Here's how the part is built. I have some questions about the finished solid (model axes, mm). A direction names the side the tool comes from. Give positions to 0.01 mm unless a question says otherwise; leave off trailing zeros. Loops run counter-clockwise (first coordinate to the right, second up) from the corner with the lowest first, then second, coordinate; pieces in that order, holes last. Notation, with made-up numbers: (46, 57) - (73, 57) arc R11 cw to (73, 73) - close; hole circle Ø7 at (18.25, 38). An arc over 180 degrees is marked (long way). Put each result on its own line as item: value. Start each with the question number.
from build123d import *

# Parameters (mm, degrees)
F0_W     = 190.5
F0_H     = 101.6
F0_W_2   = 76.2
F0_H_2   = 76.2
F1_DEPTH = 127
F2_DEPTH = 6.35
F3_R     = 5.08


with BuildPart() as f1:
    # F0 (on Top) → F1 (new body)
    with BuildSketch(Plane.XY):
        Rectangle(F0_W, F0_H)
        with Locations((-44.45, 0)):
            Rectangle(F0_W_2, F0_H_2, mode=Mode.SUBTRACT)
        with Locations((44.45, 0)):
            Rectangle(F0_W_2, F0_H_2, mode=Mode.SUBTRACT)
    extrude(amount=F1_DEPTH)

    # F0 (on Top) → F2 (join)
    with BuildSketch(Plane.XY):
        with Locations((-44.45, 0)):
            Rectangle(F0_W_2, F0_H_2)
        with Locations((44.45, 0)):
            Rectangle(F0_W_2, F0_H_2)
    extrude(amount=F2_DEPTH)

    # F3
    f3_edges = [f1.edges().sort_by_distance(p)[0] for p in [
        (-95.25, 0, 127),
        (-82.55, 0, 127),
        (-44.45, 38.1, 127),
        (-6.35, 0, 127),
        (-44.45, -38.1, 127),
        (6.35, 0, 127),
        (44.45, -38.1, 127),
        (44.45, 38.1, 127),
        (82.55, 0, 127),
        (95.25, 0, 127),
        (0, -50.8, 127),
        (0, 50.8, 127),
        (95.25, -50.8, 63.5),
        (95.25, 50.8, 63.5),
        (-95.25, -50.8, 63.5),
        (-95.25, 50.8, 63.5),
        (95.25, 0, 0),
        (0, -50.8, 0),
        (0, 50.8, 0),
        (-95.25, 0, 0),
    ]]
    fillet(f3_edges, radius=F3_R)


solid = f1.part
1) I need wall thicknesses on line 1 (X direction, y = -23.5, z = 50.5); line 2 (Y direction, x = 44.5, z = 14). Which ranges of each line are inside material? Lowest first, please.
2) Which directions (+Z, -Z, +X, -X, +Y, -Y) give clear straight access to the entire face, cutting with the end or side of a thin tool? Please do faces 4 (the cylindrical face through (-93.801, 0.64, 125.472)), 5 (the cylindrical face through (45.055, 39.628, 125.551)).
3) Suppose I cut it at C-C on y = -2. Please give me the cut outline in (x, z).
4) I'm going to push a flat-ended pin straight in: P1, Ø8, axis at x = -61, y = -28.5, coming from the +Z side. Where does the tip first touch, or does it pass through?
5) Suppose I cut it at B-B on z = 92.5. Please give me the cut outline in (x, y), plus the area to 3 significant figures.
6) Thinking about a two-plate mould opening in Y: for faces 1 (the cylindrical face through (-93.801, -49.272, 64.318)), 2 (the cylindrical face through (-84.078, 0.605, 125.551)), 3 (the cylindrical face through (-93.722, 0.64, 1.449)), which applies, pulls with the +Y half, pulls with the -Y half, needs draft (parallel to the pull), parting line crosses it, or undercut?
7) Suppose I cut it at A-A on x = 11.5. Please give me the cut outline in (y, z).
Ans:
1. line 1: x = -95.25 to -82.55, -6.35 to 6.35, 82.55 to 95.25
1. line 2: y = -50.8 to -38.1, 38.1 to 50.8
2. face 4: +Z, -X, +Y, -Y
2. face 5: +Z
3. outline: (-95.25, 5.08) arc R5.08 ccw to (-90.17, 0) - (90.17, 0) arc R5.08 ccw to (95.25, 5.08) - (95.25, 121.92) arc R5.08 ccw to (90.17, 127) - (87.63, 127) arc R5.08 ccw to (82.55, 121.92) - (82.55, 6.35) - (6.35, 6.35) - (6.35, 121.92) arc R5.08 ccw to (1.27, 127) - (-1.27, 127) arc R5.08 ccw to (-6.35, 121.92) - (-6.35, 6.35) - (-82.55, 6.35) - (-82.55, 121.92) arc R5.08 ccw to (-87.63, 127) - (-90.17, 127) arc R5.08 ccw to (-95.25, 121.92) - close
4. P1: stops at z = 6.35
5. outline: (-95.25, -45.72) arc R5.08 ccw to (-90.17, -50.8) - (90.17, -50.8) arc R5.08 ccw to (95.25, -45.72) - (95.25, 45.72) arc R5.08 ccw to (90.17, 50.8) - (-90.17, 50.8) arc R5.08 ccw to (-95.25, 45.72) - close; hole (-82.55, -38.1) - (-6.35, -38.1) - (-6.35, 38.1) - (-82.55, 38.1) - close; hole (6.35, -38.1) - (82.55, -38.1) - (82.55, 38.1) - (6.35, 38.1) - close
5. area: 7,720 mm²
6. face 1: pulls with the -Y half
6. face 2: undercut
6. face 3: needs draft
7. outline: (-50.8, 5.08) arc R5.08 ccw to (-45.72, 0) - (45.72, 0) arc R5.08 ccw to (50.8, 5.08) - (50.8, 121.92) arc R5.08 ccw to (45.72, 127) - (43.18, 127) arc R5.08 ccw to (38.1, 121.92) - (38.1, 6.35) - (-38.1, 6.35) - (-38.1, 121.92) arc R5.08 ccw to (-43.18, 127) - (-45.72, 127) arc R5.08 ccw to (-50.8, 121.92) - close
